from build123d import *

# Parameters (mm, degrees)
SKETCH2_W           = 100
SKETCH2_H           = 100
SKETCH2_R           = 4.2
BOSS_EXTRUDE1_DEPTH = 3.5
SKETCH3_R           = 4.2
CUT_EXTRUDE1_DEPTH  = 71.797245709
SKETCH4_R           = 1.6
CUT_EXTRUDE2_DEPTH  = 71.797245709


with BuildPart() as part:
    # Sketch2 → Boss-Extrude1 (new body)
    with BuildSketch(Plane(origin=(0, 0, 0), x_dir=(0, 0, -1), z_dir=(1, 0, 0))):
        Rectangle(SKETCH2_W, SKETCH2_H)
        Circle(SKETCH2_R, mode=Mode.SUBTRACT)
    extrude(amount=BOSS_EXTRUDE1_DEPTH)

    # Sketch3 → Cut-Extrude1 (cut, through all)
    with BuildSketch(Plane.ZY):
        with Locations((43.336976945, -24.938051834)):
            Circle(SKETCH3_R)
        with Locations((-43.265474881, -25.061897041)):
            Circle(SKETCH3_R)
        with Locations((-0.071502064, 49.999948875)):
            Circle(SKETCH3_R)
    extrude(amount=-CUT_EXTRUDE1_DEPTH, mode=Mode.SUBTRACT)

    # Sketch4 → Cut-Extrude2 (cut, through all)
    with BuildSketch(Plane.ZY):
        with Locations((0, -20)):
            Circle(SKETCH4_R)
    extrude(amount=-CUT_EXTRUDE2_DEPTH, mode=Mode.SUBTRACT)


solid = part.part
Design review of the part built by this model. Coordinates are the model's own, in mm. Round coordinates to 2 decimals unless told otherwise and drop trailing zeros. Write each loop counter-clockwise with the first axis right and the second up, starting at its lowest first coordinate (ties: lowest second). Pieces come first, ordered by that corner, then holes.
Item 1: Consider section A-A on z = 0. Give the boundary of the cut face in (x, y).
Item 2: Draft analysis for pull direction Y (two halves, no side actions). For faces 1 (the cylindrical face through (1.726, -18.414, -0.208)), 2 (the flat face through (2, 50, -27)), 3 (the flat face through (0, 12, 1)), 4 (the cylindrical face through (1.726, -26.547, 47.217)), state which applies: released by +Y, released by -Y, zero draft, split by the parting line, or undercut.
Item 3: Consider section B-B on z = 43.5. Give the boundary of the cut face in (x, y).
Item 4: Wall thickness on L1, parallel to Y at x = 1.7, z = 0; L2, parallel to Z at x = 0.3, y = -26.5; L3, parallel to Y at x = 1.7, z = -3: over which ranges is each line inside the solid? List them lowest first.
Item 5: Consider section C-C on x = 2.8. Give the boundary of the cut face in (y, z).
Check values:
1. outline: (0, -50) - (3.5, -50) - (3.5, -21.6) - (0, -21.6) - close; (0, -18.4) - (3.5, -18.4) - (3.5, -4.2) - (0, -4.2) - close; (0, 4.2) - (3.5, 4.2) - (3.5, 45.8) - (0, 45.8) - close
2. face 1: undercut
2. face 2: released by +Y
2. face 3: zero draft
2. face 4: undercut
3. outline: (0, -50) - (3.5, -50) - (3.5, -29.13) - (0, -29.13) - close; (0, -20.74) - (3.5, -20.74) - (3.5, 50) - (0, 50) - close
4. L1: y = -50 to -21.6, -18.4 to -4.2, 4.2 to 45.8
4. L2: z = -50 to -47.21, -39.32 to 39.44, 47.24 to 50
4. L3: y = -50 to -2.94, 2.94 to 46.99
5. outline: (-50, -50) - (50, -50) - (50, -4.27) arc R4.2 cw to (50, 4.13) - (50, 50) - (-50, 50) - close; hole circle Ø8.4 at (-25.06, -43.27); hole circle Ø8.4 at (-24.94, 43.34); hole circle Ø3.2 at (-20, 0); hole circle Ø8.4 at (0, 0)
